from build123d import *

# Parameters (mm, degrees)
SKETCH1_W               = 65
SKETCH1_H               = 30
BOSS_EXTRUDE1_DEPTH     = 3
SKETCH2_R               = 1
CUT_EXTRUDE1_DEPTH      = 5
SKETCH3_R               = 2.5
CUT_EXTRUDE2_DEPTH      = 2
SKETCH4_W               = 14.16
SKETCH4_H               = 6.4
CUT_EXTRUDE3_DEPTH      = 10
BOSS_EXTRUDE2_DEPTH     = 65
CUT_EXTRUDE4_START      = -60
CUT_EXTRUDE4_DEPTH      = 60
SKETCH7_R               = 1.5
BOSS_EXTRUDE3_DEPTH     = 3
BOSS_EXTRUDE3_2_DEPTH   = 3
CUT_EXTRUDE5_DEPTH      = 44.752699359
CUT_EXTRUDE5_DEPTH_BACK = 44.752699359
SKETCH8_R               = 6.5
CUT_EXTRUDE6_DEPTH      = 43.956940082
CUT_EXTRUDE6_DEPTH_BACK = 43.956940082
CUT_EXTRUDE7_DEPTH      = 3.175426481
CUT_EXTRUDE8_START      = 2
CUT_EXTRUDE8_DEPTH      = 3.695041823
SKETCH12_R              = 4.5
CUT_EXTRUDE9_DEPTH      = 44.752699359
SKETCH14_R              = 5.5
CUT_EXTRUDE10_DEPTH     = 43.956940082
SKETCH15_R              = 7.5
SKETCH15_R_2            = 4.5
BOSS_EXTRUDE4_DEPTH     = 8
SKETCH16_R              = 5.5
CUT_EXTRUDE11_DEPTH     = 10


# Read off the part's stored shape, not the designer's step: Cut-Extrude7, Cut-Extrude8
with BuildPart() as part:
    # Sketch1 → Boss-Extrude1 (new body)
    with BuildSketch(Plane.XY):
        Rectangle(SKETCH1_W, SKETCH1_H)
    extrude(amount=BOSS_EXTRUDE1_DEPTH)

    # Sketch2 → Cut-Extrude1 (cut)
    with BuildSketch(Plane.XY.offset(3)):
        with Locations((7.3, 11.1)):
            Circle(SKETCH2_R)
        with Locations(Location((28.7, 11.1, 0), (0, 0, 180))):
            Circle(SKETCH2_R)
        with Locations((28.7, -11.1)):
            Circle(SKETCH2_R)
        with Locations(Location((7.3, -11.1, 0), (0, 0, 180))):
            Circle(SKETCH2_R)
    extrude(amount=-CUT_EXTRUDE1_DEPTH, mode=Mode.SUBTRACT)

    # Sketch3 → Cut-Extrude2 (cut)
    with BuildSketch(Plane(origin=(0, 0, 0), x_dir=(-1, 0, 0), z_dir=(0, 0, -1))):
        with Locations((-7.3, 11.1)):
            Circle(SKETCH3_R)
        with Locations((-28.7, 11.1)):
            Circle(SKETCH3_R)
        with Locations((-28.7, -11.1)):
            Circle(SKETCH3_R)
        with Locations((-7.3, -11.1)):
            Circle(SKETCH3_R)
    extrude(amount=-CUT_EXTRUDE2_DEPTH, mode=Mode.SUBTRACT)

    # Sketch4 → Cut-Extrude3 (cut)
    with BuildSketch(Plane.XY.offset(3)):
        with Locations((18, 11.8)):
            Rectangle(SKETCH4_W, SKETCH4_H)
    extrude(amount=-CUT_EXTRUDE3_DEPTH, mode=Mode.SUBTRACT)

    # Sketch5 → Boss-Extrude2 (add)
    with BuildSketch(Plane(origin=(32.5, 0, 0), x_dir=(0, 0, -1), z_dir=(1, 0, 0))):
        Polygon((0, -15), (10, 2.320508076), (7.401923789, 3.820508076), (0, -9), align=None)
    extrude(amount=-BOSS_EXTRUDE2_DEPTH)

    # Sketch6 → Cut-Extrude4 (cut)
    with BuildSketch(Plane.XY.offset(CUT_EXTRUDE4_START)):
        with BuildLine():
            Line((8.656465997, -9), (5.943534003, -9))
            ThreePointArc((5.943534003, -9), (7.3, -13.6), (8.656465997, -9))
        make_face()
        with BuildLine():
            Line((30.056465997, -9), (27.343534003, -9))
            ThreePointArc((27.343534003, -9), (28.7, -13.6), (30.056465997, -9))
        make_face()
    extrude(amount=CUT_EXTRUDE4_DEPTH, mode=Mode.SUBTRACT)


with BuildPart() as body_2:
    # Sketch7 → Boss-Extrude3 (new body)
    with BuildSketch(Plane(origin=(0, -2.25, -3.897114317), x_dir=(1, 0, 0), z_dir=(0, 0.49999999999999445, 0.8660254037844419))):
        with BuildLine():
            Line((-35.991007953, 7.009618943), (-32.5, 7.009618943))
            Line((-32.5, 7.009618943), (-32.5, 1.009618943))
            Line((-32.5, 1.009618943), (-35.991007953, 1.009618943))
            ThreePointArc((-35.991007953, 1.009618943), (-38.991007953, 4.009618943), (-35.991007953, 7.009618943))
        make_face()
        with Locations(Location((-35.991007953, 4.009618943, 0), (0, 0, 270))):
            Circle(SKETCH7_R, mode=Mode.SUBTRACT)
    extrude(amount=-BOSS_EXTRUDE3_DEPTH)


with BuildPart() as body_3:
    # Sketch7 → Boss-Extrude3 2 (new body)
    with BuildSketch(Plane(origin=(0, -2.25, -3.897114317), x_dir=(1, 0, 0), z_dir=(0, 0.49999999999999445, 0.8660254037844419))):
        with BuildLine():
            Line((35.991007953, 7.009618943), (32.5, 7.009618943))
            Line((32.5, 7.009618943), (32.5, 1.009618943))
            Line((32.5, 1.009618943), (35.991007953, 1.009618943))
            ThreePointArc((35.991007953, 1.009618943), (38.991007953, 4.009618943), (35.991007953, 7.009618943))
        make_face()
        with Locations(Location((35.991007953, 4.009618943, 0), (0, 0, 270))):
            Circle(SKETCH7_R, mode=Mode.SUBTRACT)
    extrude(amount=-BOSS_EXTRUDE3_2_DEPTH)

    # Combine1: union part, body 2
    add(part.part)
    add(body_2.part)

    # Sketch8 → Cut-Extrude5 (cut, two sides: drawn at the far end of the back side and taken through both)
    with BuildSketch(Plane.XY.offset(3).offset(-CUT_EXTRUDE5_DEPTH_BACK)):
        with Locations(Location((-5, 7, 0), (0, 0, 180))):
            Circle(SKETCH8_R)
        with Locations(Location((-5, -7, 0), (0, 0, 270))):
            Circle(SKETCH8_R)
    extrude(amount=CUT_EXTRUDE5_DEPTH + CUT_EXTRUDE5_DEPTH_BACK, mode=Mode.SUBTRACT)

    # Sketch9 → Cut-Extrude6 (cut, two sides: drawn at the far end of the back side and taken through both)
    with BuildSketch(Plane(origin=(0, 0, 0), x_dir=(-1, 0, 0), z_dir=(0, 0, -1)).offset(-CUT_EXTRUDE6_DEPTH_BACK)):
        with BuildLine():
            Line((-1.5, 7), (-1.5, -7))
            ThreePointArc((-1.5, -7), (5, -13.5), (11.5, -7))
            Line((11.5, -7), (11.5, 7))
            ThreePointArc((11.5, 7), (5, 13.5), (-1.5, 7))
        make_face()
    extrude(amount=CUT_EXTRUDE6_DEPTH + CUT_EXTRUDE6_DEPTH_BACK, mode=Mode.SUBTRACT)

    # Cut-Extrude7 outline → Cut-Extrude7 (cut)
    with BuildSketch(Plane(origin=(0, 0, 0), x_dir=(-1, 0, 0), z_dir=(0, 0, -1))):
        with BuildLine():
            Line((-1, -13), (2.5, -13))
            ThreePointArc((2.5, -13), (0.403805922, -11.596194078), (-1, -9.5))
            Line((-1, -9.5), (-1, -13))
        make_face()
        with BuildLine():
            Line((11, -13), (11, -9.5))
            ThreePointArc((11, -9.5), (9.596194078, -11.596194078), (7.5, -13))
            Line((7.5, -13), (11, -13))
        make_face()
    extrude(amount=CUT_EXTRUDE7_DEPTH, mode=Mode.SUBTRACT)

    # Cut-Extrude8 outline → Cut-Extrude8 (cut)
    with BuildSketch(Plane(origin=(0, 0, 2), x_dir=(-1, 0, 0), z_dir=(0, 0, -1)).offset(CUT_EXTRUDE8_START)):
        with BuildLine():
            Line((-8.656465997, -9), (-5.943534003, -9))
            ThreePointArc((-5.943534003, -9), (-7.3, -8.6), (-8.656465997, -9))
        make_face()
        with BuildLine():
            Line((-30.056465997, -9), (-27.343534003, -9))
            ThreePointArc((-27.343534003, -9), (-28.7, -8.6), (-30.056465997, -9))
        make_face()
    extrude(amount=CUT_EXTRUDE8_DEPTH, mode=Mode.SUBTRACT)

    # Sketch12 → Cut-Extrude9 (cut, through all)
    with BuildSketch(Plane.XY.offset(3)):
        with Locations((-22.5, 0)):
            Circle(SKETCH12_R)
    extrude(amount=-CUT_EXTRUDE9_DEPTH, mode=Mode.SUBTRACT)

    # Sketch14 → Cut-Extrude10 (cut, through all)
    with BuildSketch(Plane(origin=(0, 0, 0), x_dir=(-1, 0, 0), z_dir=(0, 0, -1))):
        with Locations((22.5, 0)):
            Circle(SKETCH14_R)
    extrude(amount=CUT_EXTRUDE10_DEPTH, mode=Mode.SUBTRACT)

    # Sketch15 → Boss-Extrude4 (add)
    with BuildSketch(Plane.XY.offset(3)):
        with Locations((-22.5, 0)):
            Circle(SKETCH15_R)
        with Locations((-22.5, 0)):
            Circle(SKETCH15_R_2, mode=Mode.SUBTRACT)
    extrude(amount=BOSS_EXTRUDE4_DEPTH)

    # Sketch16 → Cut-Extrude11 (cut)
    with BuildSketch(Plane(origin=(0, 0, 0), x_dir=(-1, 0, 0), z_dir=(0, 0, -1))):
        with Locations((22.5, 0)):
            Circle(SKETCH16_R)
    extrude(amount=-CUT_EXTRUDE11_DEPTH, mode=Mode.SUBTRACT)


solid = body_3.part
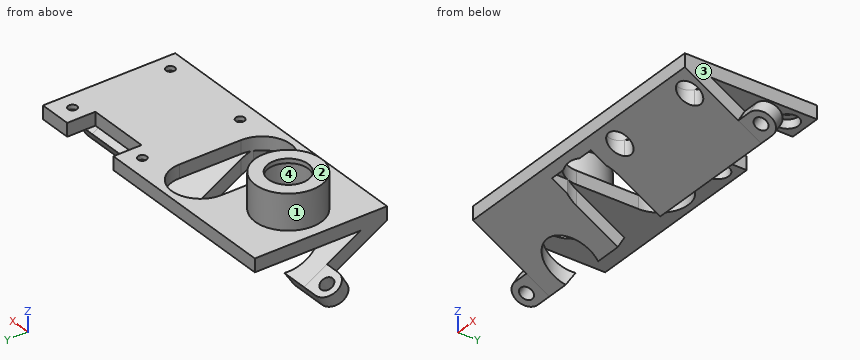
For this review, take the finished solid that the model builds, in its own axes (mm). Face numbers are marked on the shaded views. Give positions to 0.01 mm unless a question says otherwise; leave off trailing zeros. Order: outer loops, then holes, each group sorted by start corner. A loop starts at its lowest first (then second) coordinate and runs counter-clockwise, first axis right, second up. Notation, with made-up numbers: (-4.75, 34) -> (45.25, 34) arc R26 ccw to (45.25, 55) -> close; hole circle Ø1 at (27, 78.5). An arc over 180 degrees is marked (long way). Write item = value, one per line.
1) Draft analysis for pull direction X (two halves, no side actions). For the marked faces 1, 2, 3 and 4, state which applies: pulls with the +X half, pulls with the -X half, needs draft (parallel to the pull), parting line crosses it, or undercut.
Findings:
face_1 = parting line crosses it
face_2 = needs draft
face_3 = pulls with the +X half
face_4 = undercut
2) Insertion check: pin 1 (4 mm diameter, centred on x = 29.5, y = 9, fed in from -Z); pin 2 (2 mm diameter, centred on y = -0.5, z = -2, fed in from +X); pin 3 (15 mm diameter, centred on x = 3, y = -6.5, fed in from +Z); pin 4 (0.9 mm diameter, centred on x = -1.5, z = -0.5, fed in from +Y). Each pin has a flat end and moves straight along its axis. Give the tip position at first contact, or say it passes through.
Findings:
pin_1 = 0
pin_2 = through
pin_3 = 3
pin_4 = -13
3) We need section D-D, the plane x = -22.5. Give the boundary of the cut face in (y, z), and give its area (3 significant figures).
Findings:
outline = (-15, 0) -> (-5.5, -5.48) -> (-5.5, -2.02) -> (-9, 0) -> (-5.5, 0) -> (-5.5, 10) -> (-4.5, 10) -> (-4.5, 11) -> (-7.5, 11) -> (-7.5, 3) -> (-15, 3) -> close; (4.5, 10) -> (5.5, 10) -> (5.5, 0) -> (15, 0) -> (15, 3) -> (7.5, 3) -> (7.5, 11) -> (4.5, 11) -> close
area = 114 mm^2
4) We need section C-C, the plane y = 11.1. Give the boundary of the cut face in (x, z).
Findings:
outline = (-32.5, 0) -> (-10.04, 0) -> (-10.04, 3) -> (-32.5, 3) -> close; (0.04, 0) -> (4.8, 0) -> (4.8, 2) -> (6.3, 2) -> (6.3, 3) -> (0.04, 3) -> close; (8.3, 2) -> (9.8, 2) -> (9.8, 0) -> (10.92, 0) -> (10.92, 3) -> (8.3, 3) -> close; (25.08, 0) -> (26.2, 0) -> (26.2, 2) -> (27.7, 2) -> (27.7, 3) -> (25.08, 3) -> close; (29.7, 2) -> (31.2, 2) -> (31.2, 0) -> (32.5, 0) -> (32.5, 3) -> (29.7, 3) -> close
5) To check wall thickness, follow L1, parallel to X at y = -11.1, z = -0.95; L2, parallel to Y at x = 7.3, z = 2.65; L3, parallel to Y at x = -22.5, z = 7. State the ranges of each line that lie inside material, in increasing order. Write a range as from..to.
Findings:
L1 = -32.5..-11, 1..4.8, 9.8..26.2, 31.2..32.5
L2 = -15..-12.1, -10.1..10.1, 12.1..15
L3 = -7.5..-5.5, 5.5..7.5
6) We need section A-A, the plane x = 7.3. Give the boundary of the cut face in (y, z).
Findings:
outline = (-15, 0) -> (-13.6, -0.81) -> (-13.6, 2) -> (-12.1, 2) -> (-12.1, 3) -> (-15, 3) -> close; (-10.1, 2) -> (-8.6, 2) -> (-8.6, 0) -> (8.6, 0) -> (8.6, 2) -> (10.1, 2) -> (10.1, 3) -> (-10.1, 3) -> close; (-8.6, -3.7) -> (2.32, -10) -> (3.82, -7.4) -> (-8.6, -0.23) -> close; (12.1, 2) -> (13.6, 2) -> (13.6, 0) -> (15, 0) -> (15, 3) -> (12.1, 3) -> close
7) We need section B-B, the plane x = -12.5. Give the boundary of the cut face in (y, z), and give its area (3 significant figures).
Findings:
outline = (-15, 0) -> (2.32, -10) -> (3.82, -7.4) -> (-9, 0) -> (15, 0) -> (15, 3) -> (-15, 3) -> close
area = 142 mm^2
